Geometry check sheet. Reference: drawing and pictorial views, mm from the part's lowest x, y, z. A direction names the side the tool comes from. Coordinates: 2 decimals unless noted, no trailing zeros. Write each loop counter-clockwise with the first axis right and the second up, starting at its lowest first coordinate (ties: lowest second). Pieces come first, ordered by that corner, then holes. Notation, with made-up numbers: (74.25, 85.25) - (120.25, 85.25) arc R20 ccw to (120.25, 112.25) - close; hole circle Ø9 at (16.25, -10.75). An arc over 180 degrees is marked (long way). Answer as CSV lines item,"result". Start each with the question number.
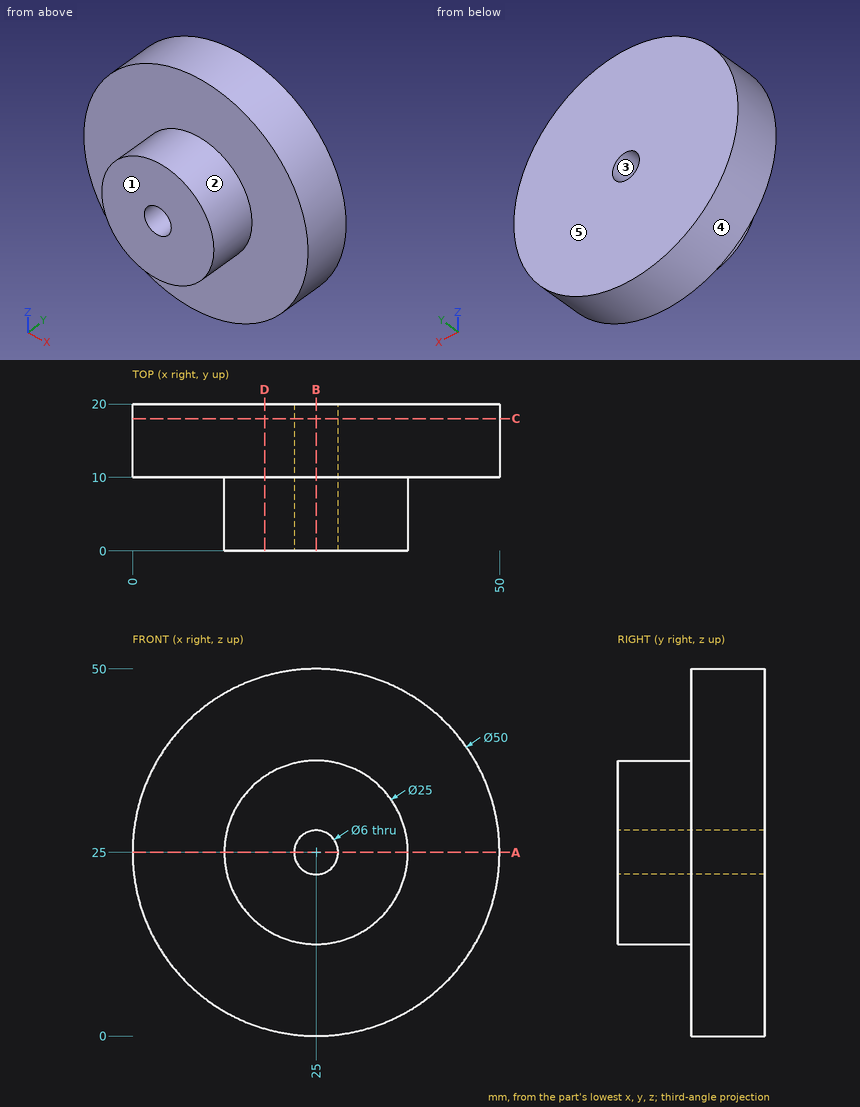
1. Access from +Z, -Z, +X, -X, +Y, -Y to the whole of each face (thin tool, end or side, straight path). Record for the marked faces 1 and 2.
2. Cross-section at B-B (x = 25). Record the cut outline in (y, z).
3. Cross-section at D-D (x = 18). Record the cut outline in (y, z).
4. Cross-section at A-A (z = 25). Record the cut outline in (x, y).
5. Depth check by flat-ended pin: P1, Ø3, axis at y = 3, z = 15, coming from the +X side; P2, Ø3, axis at y = 4.5, z = 20.5, coming from the -X side; P3, Ø3.5, axis at x = 25, z = 25, coming from the -Y side; P4, Ø6, axis at y = 9.5, z = 17.5, coming from the -X side. Enter the tip coordinate at first touch or a pass-through.
6. Draft check along Z on the marked faces 3, 4 and 5. Enter one of: pulls with the +Z half, pulls with the -Z half, needs draft (parallel to the pull), parting line crosses it, or undercut.
7. Scan lines: line 1 along Z through (x, y) = (25, 10.75); line 2 along Z through (x, y) = (25, 9.75); line 3 along Y through (x, z) = (30, 13). Record each from-to range of solid material in increasing order. Write a range as from..to.
8. Cross-section at C-C (y = 18). Record the cut outline in (x, z).
Completed:
1,face 1,"+Z, -Z, +X, -X, -Y"
1,face 2,"-Y"
2,outline,"(0, 12.5) - (10, 12.5) - (10, 0) - (20, 0) - (20, 22) - (0, 22) - close; (0, 28) - (20, 28) - (20, 50) - (10, 50) - (10, 37.5) - (0, 37.5) - close"
3,outline,"(0, 14.64) - (10, 14.64) - (10, 1) - (20, 1) - (20, 49) - (10, 49) - (10, 35.36) - (0, 35.36) - close"
4,outline,"(0, 10) - (12.5, 10) - (12.5, 0) - (22, 0) - (22, 20) - (0, 20) - close; (28, 0) - (37.5, 0) - (37.5, 10) - (50, 10) - (50, 20) - (28, 20) - close"
5,P1,"stops at x = 34.17"
5,P2,"stops at x = 12.87"
5,P3,"passes through"
5,P4,"stops at x = 0.42"
6,face 3,"undercut"
6,face 4,"parting line crosses it"
6,face 5,"needs draft"
7,line 1,"z = 0..22, 28..50"
7,line 2,"z = 12.5..22, 28..37.5"
7,line 3,"y = 10..20"
8,outline,"circle Ø50 at (25, 25); hole circle Ø6 at (25, 25)"
